Read the model definition and answer for the solid it produces. Units are mm, in the model's axes. Face numbers are marked on the shaded views. A direction names the side the tool comes from. Coordinates: 2 decimals unless noted, no trailing zeros. Write each loop counter-clockwise with the first axis right and the second up, starting at its lowest first coordinate (ties: lowest second). Pieces come first, ordered by that corner, then holes. Notation, with made-up numbers: (33.25, -5.5) -> (70.25, -5.5) arc R10 cw to (70.25, 8.5) -> close; hole circle Ø7 at (45, 82). An arc over 180 degrees is marked (long way). One line per item, written item: value. Start each with the question number.
from build123d import *

# Parameters (mm, degrees)
SKETCH1_W           = 100
SKETCH1_H           = 20
BOSS_EXTRUDE1_DEPTH = 10
SKETCH2_W           = 60
SKETCH2_H           = 20
BOSS_EXTRUDE2_DEPTH = 60
SKETCH3_R           = 10.5
CUT_EXTRUDE1_DEPTH  = 60
CUT_EXTRUDE2_START  = -20
CUT_EXTRUDE2_DEPTH  = 20
FILLET1_R           = 2.54
FILLET2_R           = 2.54


# Read off the part's stored shape, not the designer's step: Cut-Extrude2
with BuildPart() as part:
    # Sketch1 → Boss-Extrude1 (new body)
    with BuildSketch(Plane(origin=(0, 0, 0), x_dir=(1, 0, 0), z_dir=(0, 1, 0))):
        with Locations((0.812697448, -5.425302539)):
            Rectangle(SKETCH1_W, SKETCH1_H)
    extrude(amount=BOSS_EXTRUDE1_DEPTH)

    # Sketch2 → Boss-Extrude2 (add)
    with BuildSketch(Plane(origin=(0, 10, 0), x_dir=(1, 0, 0), z_dir=(0, 1, 0))):
        with Locations((0.812697448, -5.425302539)):
            Rectangle(SKETCH2_W, SKETCH2_H)
    extrude(amount=BOSS_EXTRUDE2_DEPTH)

    # Sketch3 → Cut-Extrude1 (cut)
    with BuildSketch(Plane.XY.offset(15.425302539)):
        with Locations((0.812697448, 54.837920596)):
            Circle(SKETCH3_R)
    extrude(amount=-CUT_EXTRUDE1_DEPTH, mode=Mode.SUBTRACT)

    # Cut-Extrude2 outline → Cut-Extrude2 (cut)
    with BuildSketch(Plane.XY.offset(15.425302539).offset(CUT_EXTRUDE2_START)):
        with BuildLine():
            Line((-29.187302552, 10), (-14.985674084, 57.602633157))
            add(Edge.make_bspline(
                [(-14.985674084, 57.602633157), (-13.129301822, 64.096984003), (-6.152391174, 70.000002699), (0.804550116, 70.000002699)],
                knots=[0, 0, 0, 0, 0.498740566, 0.498740566, 0.498740566, 0.498740566], degree=3))
            Line((0.804550116, 70.000002699), (-29.187302552, 70))
            Line((-29.187302552, 70), (-29.187302552, 10))
        make_face()
        with BuildLine():
            Line((30.812697448, 70), (0.80589599, 70.000002625))
            add(Edge.make_bspline(
                [(0.80589599, 70.000002625), (0.808163145, 70.000002377), (7.799782278, 69.997303833), (14.769205665, 64.030481045), (16.767488499, 57.602633157)],
                knots=[0.498772728, 0.498772728, 0.498772728, 0.498772728, 0.49893526, 1, 1, 1, 1], degree=3))
            Line((16.767488499, 57.602633157), (30.812697448, 10))
            Line((30.812697448, 10), (30.812697448, 70))
        make_face()
    extrude(amount=CUT_EXTRUDE2_DEPTH, mode=Mode.SUBTRACT)

    # Fillet1
    fillet1_edges = [part.edges().sort_by_distance(p)[0] for p in [
        (-29.187302552, 10, 5.425302539),
    ]]
    fillet(fillet1_edges, radius=FILLET1_R)

    # Fillet2
    fillet2_edges = [part.edges().sort_by_distance(p)[0] for p in [
        (30.812697448, 10, 5.425302539),
    ]]
    fillet(fillet2_edges, radius=FILLET2_R)


solid = part.part
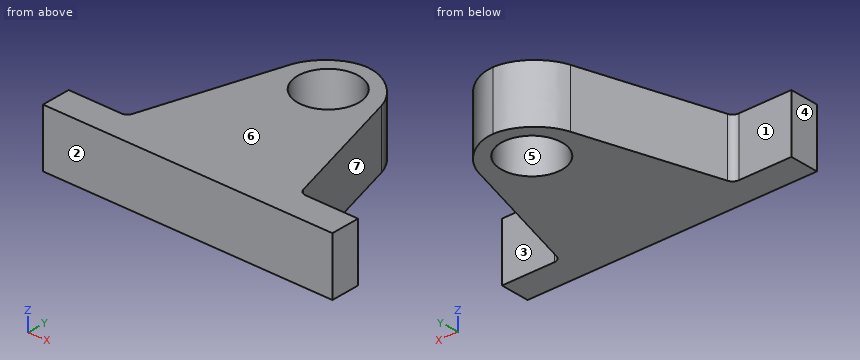
1. A tool of negligible diameter and unlimited length cuts with its end or side. For the marked faces 1, 2 and 3, from which of +Z, -Z, +X, -X, +Y, -Y can it reach the whole face along a straight path? Write none if from no direction.
2. For a pull along X with two mould halves and no side action, classify the marked faces 4, 5, 6 and 7 as +X half, -X half, draft (parallel to the pull), parting line (faces both ways), or undercut.
3. A cutting plane is placed at A-A on y = 50. Give the vertices of the cut face in (x, z), then the cut area to 3 significant figures.
4. A cutting plane is placed at C-C on y = 33. Give the vertices of the cut face in (x, z).
5. Find the intervals of material crossed by probe 1 along Y at (x, z) = (1, 6.25); probe 2 along Y at (x, z) = (-42, 7); probe 3 along Y at (x, z) = (-3.5, 10.5), in increasing order. Write a range as from..to.
6. Given pin 1 (1.5 mm diameter, centred on y = 41.5, z = 6.5, fed in from +X); pin 2 (3 mm diameter, centred on y = 21, z = -1, fed in from -X); pin 3 (8 mm diameter, centred on x = -1.5, z = -1, fed in from +Y); pin 4 (3 mm diameter, centred on x = -31.5, z = 1, fed in from +Y), each flat-ended and moving along its own axis, determine where each tip first touches the part or whether it passes through.
7. A cutting plane is placed at B-B on x = -39. Give the vertices of the cut face in (y, z), then the cut area to 3 significant figures.
Derived:
1. face 1: +Z, -Z, -X, +Y
1. face 2: +Z, -Z, +X, -X, -Y
1. face 3: +Z, -Z, +X, +Y
2. face 4: -X half
2. face 5: undercut
2. face 6: draft
2. face 7: +X half
3. outline: (-17.25, -4.57) -> (-8.51, -4.57) -> (-8.51, 15.43) -> (-17.25, 15.43) -> close; (10.13, -4.57) -> (19.01, -4.57) -> (19.01, 15.43) -> (10.13, 15.43) -> close
3. area: 353 mm2
4. outline: (-22.33, -4.57) -> (24.03, -4.57) -> (24.03, 15.43) -> (-22.33, 15.43) -> close
5. probe 1: y = 0..44.34, 65.34..70
5. probe 2: y = 0..10
5. probe 3: y = 0..45.26, 64.41..69.28
6. pin 1: stops at x = 21.74
6. pin 2: stops at x = -26.35
6. pin 3: stops at y = 70
6. pin 4: stops at y = 10.24
7. outline: (0, -4.57) -> (10, -4.57) -> (10, 15.43) -> (0, 15.43) -> close
7. area: 200 mm2
